Model file for the job. Use its own axes, mm. Face numbers are marked on the shaded views. A direction names the side the tool comes from. Round coordinates to 2 decimals unless told otherwise and drop trailing zeros. Loops run counter-clockwise (first coordinate to the right, second up) from the corner with the lowest first, then second, coordinate; pieces in that order, holes last. Notation, with made-up numbers: (-36.5, 61.25) - (-27.5, 61.25) arc R19 cw to (-27.5, 84.25) - close; hole circle Ø6 at (42.25, 9.5). An arc over 180 degrees is marked (long way). Answer as a JSON object with one key per item and string values.
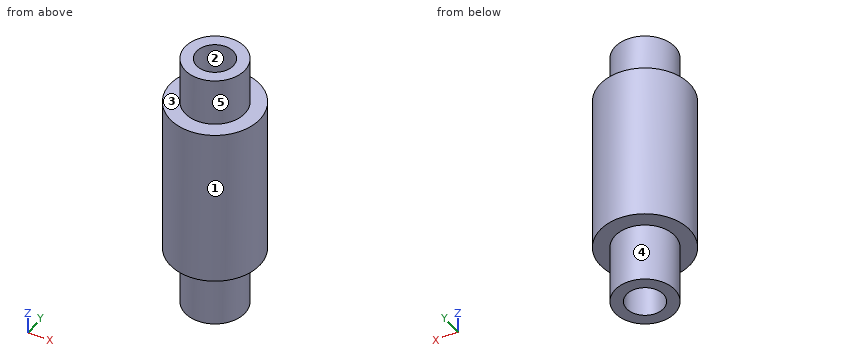
Autodesk Inventor part; units mm, degrees
ref_plane "YZ Plane" through (0, 0, 0) normal (1, 0, 0) x (0, 1, 0)
ref_plane "XZ Plane" through (0, 0, 0) normal (0, 1, 0) x (-1, 0, 0)
ref_plane "XY Plane" through (0, 0, 0) normal (0, 0, 1) x (1, 0, 0)
sketch "スケッチ1" plane through (0, 0, 0) normal (0, 0, 1) x (1, 0, 0)
  circle A0 centre (0, 0) radius 3
  dimension "d0" = 6
extrude "押し出し1" add sketch "スケッチ1" along normal blind 18
sketch "スケッチ3" plane through (0, 0, 18) normal (0, 0, 1) x (1, 0, 0)
  circle A0 centre (0, 0) radius 3
hole "Hole2" at (0, 0, 18) direction (0, 0, -1) diameter 2.459 end through all
sketch "スケッチ4" plane through (0, 0, 18) normal (0, 0, 1) x (1, 0, 0)
  circle A0 centre (0, 0) radius 3
  circle A1 centre (0, 0) radius 2
  dimension "d20" = 4
extrude "押し出し2" cut sketch "スケッチ4" against normal blind 3.2
sketch "スケッチ5" plane through (0, 0, 0) normal (0, 0, -1) x (-1, 0, 0)
  circle A0 centre (0, 0) radius 3
  circle A1 centre (0, 0) radius 2
  dimension "d23" = 4
extrude "押し出し3" cut sketch "スケッチ5" against normal blind 4
properties part number "shaft6-19"
1) Tool access for the marked faces 4 and 5: list every direction of +Z, -Z, +X, -X, +Y, -Y with a clear straight run to the whole face (end or side of a thin tool).
Values follow:
{"face 4": "-Z", "face 5": "+Z"}
2) Slice it at A-A on y = 0. List the corners of the cut face in (x, z).
Values follow:
{"outline": "(-3, 4) - (-2, 4) - (-2, 0) - (-1.23, 0) - (-1.23, 18) - (-2, 18) - (-2, 14.8) - (-3, 14.8) - close; (1.23, 0) - (2, 0) - (2, 4) - (3, 4) - (3, 14.8) - (2, 14.8) - (2, 18) - (1.23, 18) - close"}
3) Slice it at C-C on z = 13.25. List the corners of the cut face in (x, y).
Values follow:
{"outline": "circle Ø6 at (0, 0); hole circle Ø2.46 at (0, 0)"}
4) Probe probe 1 along Y at (x, z) = (0, 9.5); probe 2 along Z at (x, y) = (1.75, -2.1); probe 3 along X at (y, z) = (-0.4, 9). List the from-to ranges inside material, lowest first.
Values follow:
{"probe 1": "-3 to -1.23, 1.23 to 3", "probe 2": "4 to 14.8", "probe 3": "-2.97 to -1.16, 1.16 to 2.97"}
5) Drop flat-ended pins along their axis: P1, Ø2, axis at x = 0, y = 1, coming from the -Z side; P2, Ø1.5, axis at x = -2, z = 14.5, coming from the +Y side; P3, Ø2, axis at x = 0, y = 0, coming from the +Z side. Give the stop position or say it passes through.
Values follow:
{"P1": "z = 0", "P2": "y = 2.73", "P3": "through"}
6) Two-plate mould, pull along X, no slides. Class the marked faces 1, 2 and 3: pulls with the +X half, pulls with the -X half, needs draft (parallel to the pull), parting line crosses it, or undercut.
Values follow:
{"face 1": "parting line crosses it", "face 2": "undercut", "face 3": "needs draft"}
7) Slice it at D-D on y = -1.7. List the corners of the cut face in (x, z).
Values follow:
{"outline": "(-2.47, 4) - (-1.05, 4) - (-1.05, 0) - (1.05, 0) - (1.05, 4) - (2.47, 4) - (2.47, 14.8) - (1.05, 14.8) - (1.05, 18) - (-1.05, 18) - (-1.05, 14.8) - (-2.47, 14.8) - close"}
